from build123d import *

# Parameters (mm, degrees)
F0_R     = 10
F1_DEPTH = 3
F2_R     = 7.5
F3_DEPTH = 5
F4_W     = 6.5
F4_H     = 2
F4_W_2   = 2
F4_H_2   = 6.5
F5_DEPTH = 1


with BuildPart() as f1:
    # F0 (on Top) → F1 (new body)
    with BuildSketch(Plane.XY):
        Circle(F0_R)
    extrude(amount=F1_DEPTH)

    # F2 (on face) → F3 (join)
    with BuildSketch(Plane.XY.offset(3)):
        Circle(F2_R)
    extrude(amount=F3_DEPTH)

    # F4 (on face) → F5 (cut)
    with BuildSketch(Plane(origin=(0, 0, 0), x_dir=(1, 0, 0), z_dir=(0, 0, -1))):
        with Locations((4.25, 0)):
            Rectangle(F4_W, F4_H)
        with Locations((0, -4.25)):
            Rectangle(F4_W_2, F4_H_2)
        Rectangle(F4_W_2, F4_H)
        with Locations((-4.25, 0)):
            Rectangle(F4_W, F4_H)
        with Locations((0, 4.25)):
            Rectangle(F4_W_2, F4_H_2)
    extrude(amount=-F5_DEPTH, mode=Mode.SUBTRACT)


solid = f1.part
Model file for the job. Use its own axes, mm. A direction names the side the tool comes from. Round coordinates to 2 decimals unless told otherwise and drop trailing zeros. Loops run counter-clockwise (first coordinate to the right, second up) from the corner with the lowest first, then second, coordinate; pieces in that order, holes last.
1. Band-saw the part on A-A, the plane x = 0. List the corners of the cut face in (y, z), and give its area (3 significant figures).
Check values:
outline: (-10, 0) - (-7.5, 0) - (-7.5, 1) - (7.5, 1) - (7.5, 0) - (10, 0) - (10, 3) - (7.5, 3) - (7.5, 8) - (-7.5, 8) - (-7.5, 3) - (-10, 3) - close
area: 120 mm2
2. Wall check: probe 1 along Z at (x, y) = (-8.75, 3); probe 2 along X at (y, z) = (-0.25, 5); probe 3 along X at (y, z) = (-4.5, 0.75). Give the ranges that are in metal, low to high.
Check values:
probe 1: z = 0 to 3
probe 2: x = -7.5 to 7.5
probe 3: x = -8.93 to -1, 1 to 8.93
3. Tool access for faces 4 (the cylindrical face through (-7.493, 0.33, 5.465)), 5 (the flat face through (0, 0, 8)), 6 (the flat face through (4.3, -1, 0.5)): list every direction of +Z, -Z, +X, -X, +Y, -Y with a clear straight run to the whole face (end or side of a thin tool).
Check values:
face 4: +Z
face 5: +Z, +X, -X, +Y, -Y
face 6: -Z
4. Drop flat-ended pins along their axis: P1, Ø12, axis at x = 3, y = -3, coming from the -Z side; P2, Ø0.8, axis at y = -4, z = 0.5, coming from the -X side; P3, Ø0.5, axis at y = -5.5, z = 0.5, coming from the +X side; P4, Ø1.1, axis at x = -5, z = 0.5, coming from the +Y side. Give the stop position or say it passes through.
Check values:
P1: stops at z = 0
P2: stops at x = -9.33
P3: stops at x = 8.51
P4: stops at y = 8.96
5. Band-saw the part on D-D, the plane x = -8. List the corners of the cut face in (y, z).
Check values:
outline: (-6, 0) - (6, 0) - (6, 3) - (-6, 3) - close
6. Mould opens along Y. For faces 1 (the flat face through (0, -7.5, 0.5)), 2 (the flat face through (2, -2, 0)), 3 (the cylindrical face through (-2.17, -9.76, 1.48)) say: +Y half, -Y half, draft (parallel to the pull), parting line (faces both ways), or undercut.
Check values:
face 1: undercut
face 2: draft
face 3: parting line
7. Band-saw the part on C-C, the plane z = 4. List the corners of the cut face in (x, y).
Check values:
outline: circle Ø15 at (0, 0)
